The listing builds one solid part. Answer for the finished solid, in the listing's coordinates (mm). Face numbers are marked on the shaded views. A direction names the side the tool comes from. Round coordinates to 2 decimals unless told otherwise and drop trailing zeros. Write each loop counter-clockwise with the first axis right and the second up, starting at its lowest first coordinate (ties: lowest second). Pieces come first, ordered by that corner, then holes. Notation, with made-up numbers: M 9,84.25 L 19,84.25 A25 cw 19,110.25 Z; hole C -12,-19.75 d3. An arc over 180 degrees is marked long. Write each question's results on one line, items separated by ' | '.
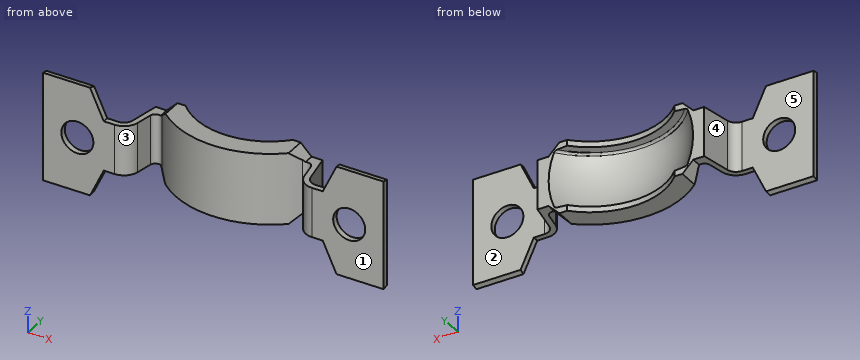
Solid Edge part; units mm, degrees
sketch "Sketch1" plane through (0, 0, 0) normal (0, 0, 1) x (1, 0, 0)
  line L0 (-59.5, -31) -> (-59.5, -33)
  line L1 (-59.5, -33) -> (-34.5, -33)
  arc A0 (-34.5, -33) -> (-29.0964, -28.5251) centre (-34.5, -27.5) ccw
  line L2 (-29.0964, -28.5251) -> (-28.0428, -22.9713)
  arc A1 (-28.0428, -22.9713) -> (-24.5877, -22.0101) centre (-26.0779, -23.3441) cw
  arc A2 (-24.5877, -22.0101) -> (24.5877, -22.0101) centre (0, 0) ccw
  arc A3 (24.5877, -22.0101) -> (28.0428, -22.9713) centre (26.0779, -23.3441) cw
  line L3 (28.0428, -22.9713) -> (29.0964, -28.5251)
  arc A4 (29.0964, -28.5251) -> (34.5, -33) centre (34.5, -27.5) ccw
  line L4 (34.5, -33) -> (59.5, -33)
  line L5 (59.5, -33) -> (59.5, -31)
  line L6 (59.5, -31) -> (34.5, -31)
  arc A5 (34.5, -31) -> (31.0613, -28.1523) centre (34.5, -27.5) cw
  line L7 (31.0613, -28.1523) -> (28.2379, -13.2688)
  arc A6 (28.2379, -13.2688) -> (-28.2379, -13.2688) centre (0, 0) cw
  line L8 (-28.2379, -13.2688) -> (-31.0613, -28.1523)
  arc A7 (-31.0613, -28.1523) -> (-34.5, -31) centre (-34.5, -27.5) cw
  line L9 (-34.5, -31) -> (-59.5, -31)
extrude "ExtrudedProtrusion_1" add sketch "Sketch1" against normal blind 19 and the other way blind 19
sketch "Sketch2" plane through (0, 0, 0) normal (1, 0, 0) x (0, 1, 0)
  line L0 (-33, 19) -> (0, 12.5)
  line L1 (0, 12.5) -> (33, 12.5)
  line L2 (33, 12.5) -> (33, -12.5)
  line L3 (33, -12.5) -> (0, -12.5)
  line L4 (0, -12.5) -> (-33, -19)
  line L5 (-33, -19) -> (34, -19)
  line L6 (34, -19) -> (34, 19)
  line L7 (34, 19) -> (-33, 19)
extrude "ExtrudedCutout_1" cut sketch "Sketch2" against normal blind 59.5 and the other way blind 59.5
hole "Hole_1" at (47.5, 0, 0) direction (0, -1, 0) diameter 11.2 depth 33
hole "Hole_2" at (-47.5, 0, 0) direction (0, -1, 0) diameter 11.2 depth 33
sketch "Sketch3" plane through (0, 0, 0) normal (1, 0, 0) x (0, 1, 0)
  line L0 (-26, 12.5) -> (-31.35, 12.5)
  line L1 (-31.35, 12.5) -> (-31.35, -12.5)
  line L2 (-31.35, -12.5) -> (-26, -12.5)
  line L3 (-26, -12.5) -> (-26, -10.5)
  line L4 (-26, -10.5) -> (-28.6598, -10.207)
  arc A0 (-28.6598, -10.207) -> (-29.502, -9.5201) centre (-28.5503, -9.213) cw
  arc A1 (-29.502, -9.5201) -> (-29.502, 9.5201) centre (0, 0) cw
  arc A2 (-29.502, 9.5201) -> (-28.6598, 10.207) centre (-28.5503, 9.213) cw
  line L5 (-28.6598, 10.207) -> (-26, 10.5)
  line L6 (-26, 10.5) -> (-26, 12.5)
revolve "RevolvedProtrusion1" add sketch "Sketch3" angle 360 about axis through (0, 0, 19) along (0, 0, -1)
sketch "Sketch4" plane through (0, 0, 0) normal (1, 0, 0) x (0, 1, 0)
  line L0 (48, 38) -> (-18, 38)
  line L1 (-18, 38) -> (-18, -38)
  line L2 (-18, -38) -> (48, -38)
  line L3 (48, -38) -> (48, 38)
extrude "ExtrudedCutout_2" cut sketch "Sketch4" against normal blind 119 and the other way blind 119
sketch "Sketch5" plane through (0, 0, 0) normal (0, -1, 0) x (1, 0, 0)
  line L0 (-69.5, 29) -> (69.5, 29)
  line L1 (69.5, 29) -> (69.5, -29)
  line L2 (69.5, -29) -> (-69.5, -29)
  line L3 (-69.5, -29) -> (-69.5, 29)
  line L4 (-59.5, -19) -> (-59.5, 19)
  line L5 (-59.5, 19) -> (-43.0643, 19)
  line L6 (-43.0643, 19) -> (-38.2614, 8.7)
  line L7 (-38.2614, 8.7) -> (-25.3, 8.7)
  line L8 (-25.3, 8.7) -> (-21.5, 12.5)
  line L9 (-21.5, 12.5) -> (21.5, 12.5)
  line L10 (21.5, 12.5) -> (25.3, 8.7)
  line L11 (25.3, 8.7) -> (38.2614, 8.7)
  line L12 (38.2614, 8.7) -> (43.0643, 19)
  line L13 (43.0643, 19) -> (59.5, 19)
  line L14 (59.5, 19) -> (59.5, -19)
  line L15 (59.5, -19) -> (43.0643, -19)
  line L16 (43.0643, -19) -> (38.2614, -8.7)
  line L17 (38.2614, -8.7) -> (25.3, -8.7)
  line L18 (25.3, -8.7) -> (21.5, -12.5)
  line L19 (21.5, -12.5) -> (-21.5, -12.5)
  line L20 (-21.5, -12.5) -> (-25.3, -8.7)
  line L21 (-25.3, -8.7) -> (-38.2614, -8.7)
  line L22 (-38.2614, -8.7) -> (-43.0643, -19)
  line L23 (-43.0643, -19) -> (-59.5, -19)
extrude "ExtrudedCutout_3" cut sketch "Sketch5" along normal blind 33
properties part number "housingP 62-h"
1) A tool of negligible diameter and unlimited length cuts with its end or side. For the marked faces 1 and 2, from which of +Z, -Z, +X, -X, +Y, -Y can it reach the whole face along a straight path? Write none if from no direction.
Return value:
face 1: +Z, -Z, +X, -X, -Y | face 2: +Z, -Z, +X, +Y
2) Each of these flat-tipped pins is pushed along its axis until it touches: pin 1 (13 mm diameter, centred on x = 47.5, z = 0, fed in from +Y); pin 2 (7.5 mm diameter, centred on x = 5.5, y = -23.5, fed in from +Z); pin 3 (6 mm diameter, centred on y = -21, z = 6.5, fed in from +X). Where does it stop, or does it pass through?
Return value:
pin 1: y = -31 | pin 2: z = 12.5 | pin 3: x = 30.27
3) Section A-A (x = 47.5) is taken. Determine the outline of the cut face in (y, z).
Return value:
outline: M -33,-19 L -31,-18.61 L -31,-5.6 L -33,-5.6 Z; M -33,5.6 L -31,5.6 L -31,18.61 L -33,19 Z
4) Find the intervals of material crossed by line 1 (X direction, y = -23.25, z = -5); line 2 (X direction, y = -19.5, z = 7); line 3 (Y direction, x = -52, z = 15), in increasing order.
Return value:
line 1: -30.13 to -28.1, -23.42 to -19.89, 19.89 to 23.42, 28.1 to 30.13 | line 2: -29.42 to -23.06, 23.06 to 29.42 | line 3: -33 to -31
5) The mould has two halves that part along X. Classify the marked faces 3, 4 and 5: +X half, -X half, draft (parallel to the pull), parting line (faces both ways), or undercut.
Return value:
face 3: undercut | face 4: -X half | face 5: draft
6) Section B-B (z = -0.5) is taken. Determine the outline of the cut face in (x, y).
Return value:
outline: M -59.5,-33 L -53.08,-33 L -53.08,-31 L -59.5,-31 Z; M -41.92,-33 L -34.5,-33 A5.5 ccw -29.1,-28.53 L -28.04,-22.97 A2 cw -24.59,-22.01 A33 ccw 24.59,-22.01 A2 cw 28.04,-22.97 L 29.1,-28.53 A5.5 ccw 34.5,-33 L 41.92,-33 L 41.92,-31 L 34.5,-31 A3.5 cw 31.06,-28.15 L 29.14,-18 L 25.23,-18 A31 cw -25.23,-18 L -29.14,-18 L -31.06,-28.15 A3.5 cw -34.5,-31 L -41.92,-31 Z; M 53.08,-33 L 59.5,-33 L 59.5,-31 L 53.08,-31 Z
